Work out the finished part from the listing and answer in its coordinate system (mm). Face numbers are marked on the shaded views. A direction names the side the tool comes from. Coordinates: 2 decimals unless noted, no trailing zeros. Order: outer loops, then holes, each group sorted by start corner. A loop starts at its lowest first (then second) coordinate and runs counter-clockwise, first axis right, second up. Notation, with made-up numbers: M -26.75,77.25 L -5.75,77.25 A20 cw -5.75,112.25 Z; hole C -40,17 d9. An arc over 180 degrees is marked long. Write item = value, one per line. Start each with the question number.
Q1. Each of these flat-tipped pins is pushed along its axis until it touches: P1, Ø11.5, axis at x = 54, z = -9, coming from the +Y side; P2, Ø6, axis at x = 16, y = -27.5, coming from the +Z side; P3, Ø13.5, axis at y = -37, z = -27.5, coming from the +X side; P4, Ø6, axis at y = -57.5, z = 64.5, coming from the +X side. Where does it stop, or does it pass through?
Q2. Find section A-A on z = -41. Give the vertices of the cut face in (x, y).
Q3. Straight lines are drawn through the part: line 1 along Y through (x, z) = (-31, 3); line 2 along Z through (x, y) = (-23, -27.5); line 3 along Y through (x, z) = (42, 14). For each, find the intervals that lie inside material, in ascending order.
Q4. A tool of negligible diameter and unlimited length cuts with its end or side. For the marked faces 1, 2, 3, 4 and 5, from which of +Z, -Z, +X, -X, +Y, -Y can it reach the whole face along a straight path? Write none if from no direction.
Q5. Determine the mould class of the marked faces 6, 7 and 8 for opening direction Y: released by +Y, released by -Y, zero draft, split by the parting line, or undercut.
Q6. Find section B-B on x = -48. Give the vertices of the cut face in (y, z), and give its area (3 significant figures).
Q7. Find section C-C on y = -101.5. Give the vertices of the cut face in (x, z), and give its area (3 significant figures).
Q8. Find section D-D on z = 0. Give the vertices of the cut face in (x, y) (1 decimal), and give its area (3 significant figures).
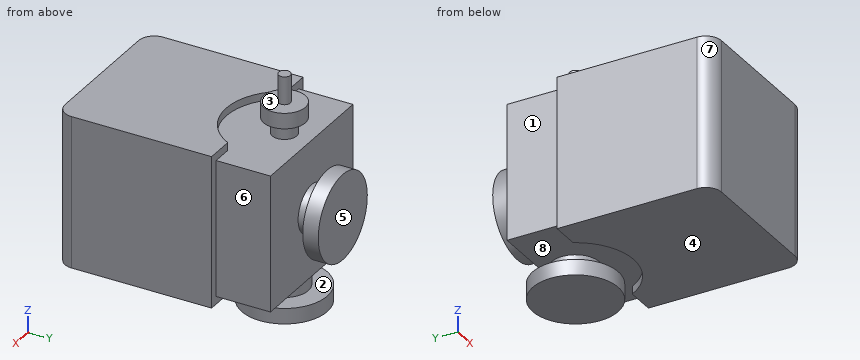
```python
from build123d import *

# Parameters (mm, degrees)
SKETCH1_R           = 34.925
BOSS_EXTRUDE1_DEPTH = 12.69
SKETCH2_R           = 19.4
BOSS_EXTRUDE2_DEPTH = 12.69
SKETCH7_W           = 117.475
SKETCH7_H           = 111.125
BOSS_EXTRUDE3_DEPTH = 44.45
SKETCH8_W           = 130.175
SKETCH8_H           = 123.825
BOSS_EXTRUDE4_DEPTH = 127
FILLET1_R           = 12.7
FILLET2_R           = 12.7
SKETCH9_R           = 47.625
CUT_EXTRUDE1_DEPTH  = 228.91291732
SKETCH10_R          = 19.4
BOSS_EXTRUDE5_DEPTH = 12.7
SKETCH11_R          = 34.925
BOSS_EXTRUDE6_DEPTH = 12.7
SKETCH17_R          = 47.625
CUT_EXTRUDE3_DEPTH  = 239.291833434
SKETCH13_R          = 10
BOSS_EXTRUDE7_DEPTH = 12.7
SKETCH14_R          = 17.018
BOSS_EXTRUDE8_DEPTH = 12.7
SKETCH15_R          = 4.785590778
BOSS_EXTRUDE9_DEPTH = 22.7


with BuildPart() as part:
    # Sketch1 → Boss-Extrude1 (new body)
    with BuildSketch(Plane(origin=(0, 0, 0), x_dir=(1, 0, 0), z_dir=(0, 1, 0))):
        with Locations(Location((0, 0, 0), (0, 0, 270))):
            Circle(SKETCH1_R)
    extrude(amount=BOSS_EXTRUDE1_DEPTH)

    # Sketch2 → Boss-Extrude2 (add)
    with BuildSketch(Plane(origin=(0, 0, 0), x_dir=(-1, 0, 0), z_dir=(0, -1, 0))):
        with Locations(Location((0, 0, 0), (0, 0, 90))):
            Circle(SKETCH2_R)
    extrude(amount=BOSS_EXTRUDE2_DEPTH)

    # Sketch7 → Boss-Extrude3 (add)
    with BuildSketch(Plane.XZ.offset(12.69)):
        Rectangle(SKETCH7_W, SKETCH7_H)
    extrude(amount=BOSS_EXTRUDE3_DEPTH)

    # Sketch8 → Boss-Extrude4 (add)
    with BuildSketch(Plane.XZ.offset(57.14)):
        Rectangle(SKETCH8_W, SKETCH8_H)
    extrude(amount=BOSS_EXTRUDE4_DEPTH)

    # Fillet1
    fillet1_edges = [part.edges().sort_by_distance(p)[0] for p in [
        (65.0875, -184.14, 0),
    ]]
    fillet(fillet1_edges, radius=FILLET1_R)

    # Fillet2
    fillet2_edges = [part.edges().sort_by_distance(p)[0] for p in [
        (-65.0875, -184.14, 0),
    ]]
    fillet(fillet2_edges, radius=FILLET2_R)

    # Sketch9 → Cut-Extrude1 (cut, through all)
    with BuildSketch(Plane(origin=(0, 0, -55.5625), x_dir=(-1, 0, 0), z_dir=(0, 0, -1))):
        with Locations((0, -34.915)):
            Circle(SKETCH9_R)
    extrude(amount=CUT_EXTRUDE1_DEPTH, mode=Mode.SUBTRACT)

    # Sketch10 → Boss-Extrude5 (add)
    with BuildSketch(Plane(origin=(0, 0, -55.5625), x_dir=(-1, 0, 0), z_dir=(0, 0, -1))):
        with Locations(Location((0, -34.915, 0), (0, 0, 180))):
            Circle(SKETCH10_R)
    extrude(amount=BOSS_EXTRUDE5_DEPTH)

    # Sketch11 → Boss-Extrude6 (add)
    with BuildSketch(Plane(origin=(0, 0, -68.2625), x_dir=(-1, 0, 0), z_dir=(0, 0, -1))):
        with Locations((0, -34.915)):
            Circle(SKETCH11_R)
    extrude(amount=BOSS_EXTRUDE6_DEPTH)

    # Sketch17 → Cut-Extrude3 (cut, through all)
    with BuildSketch(Plane.XY.offset(55.5625)):
        with Locations((0, -34.915)):
            Circle(SKETCH17_R)
    extrude(amount=CUT_EXTRUDE3_DEPTH, mode=Mode.SUBTRACT)

    # Sketch13 → Boss-Extrude7 (add)
    with BuildSketch(Plane.XY.offset(55.5625)):
        with Locations(Location((0, -34.915, 0), (0, 0, 180))):
            Circle(SKETCH13_R)
    extrude(amount=BOSS_EXTRUDE7_DEPTH)

    # Sketch14 → Boss-Extrude8 (add)
    with BuildSketch(Plane.XY.offset(68.2625)):
        with Locations((0, -34.915)):
            Circle(SKETCH14_R)
    extrude(amount=BOSS_EXTRUDE8_DEPTH)

    # Sketch15 → Boss-Extrude9 (add)
    with BuildSketch(Plane.XY.offset(80.9625)):
        with Locations((0, -34.915)):
            Circle(SKETCH15_R)
    extrude(amount=BOSS_EXTRUDE9_DEPTH)


solid = part.part
```
Findings below:
q1.P1 = -12.69
q1.P2 = 80.96
q1.P3 = 58.74
q1.P4 = 65.09
q2.outline = M -65.09,-171.44 A12.7 ccw -52.39,-184.14 L 52.39,-184.14 A12.7 ccw 65.09,-171.44 L 65.09,-57.14 L 58.74,-57.14 L 58.74,-12.69 L -58.74,-12.69 L -58.74,-57.14 L -65.09,-57.14 Z
q3.line_1 = -184.14 to -12.69, 0 to 12.69
q3.line_2 = -80.96 to -68.26, -55.56 to 55.56
q3.line_3 = -184.14 to -12.69
q4.face_1 = +Z, -Z, -X, +Y
q4.face_2 = none
q4.face_3 = +Z
q4.face_4 = -Z, +X, -X, -Y
q4.face_5 = +Z, -Z, +X, -X, +Y
q5.face_6 = zero draft
q5.face_7 = released by -Y
q5.face_8 = undercut
q6.outline = M -184.14,-61.91 L -57.14,-61.91 L -57.14,-55.56 L -12.69,-55.56 L -12.69,55.56 L -57.14,55.56 L -57.14,61.91 L -184.14,61.91 Z
q6.area = 20,700 mm^2
q7.outline = M -65.09,-61.91 L 65.09,-61.91 L 65.09,61.91 L -65.09,61.91 Z
q7.area = 16,100 mm^2
q8.outline = M -65.1,-171.4 A12.7 ccw -52.4,-184.1 L 52.4,-184.1 A12.7 ccw 65.1,-171.4 L 65.1,-57.1 L 58.7,-57.1 L 58.7,-12.7 L 19.4,-12.7 L 19.4,0 L 34.9,0 L 34.9,12.7 L -34.9,12.7 L -34.9,0 L -19.4,0 L -19.4,-12.7 L -58.7,-12.7 L -58.7,-57.1 L -65.1,-57.1 Z
q8.area = 23,100 mm^2
